For this review, take the finished solid that the model builds, in its own axes (mm). Coordinates: 2 decimals unless noted, no trailing zeros. Write each loop counter-clockwise with the first axis right and the second up, starting at its lowest first coordinate (ties: lowest second). Pieces come first, ordered by that corner, then holes.
1) We need section B-B on z = 1.9. Give the number of separate pieces and of enclosed holes in the cut face, then the cut area to 3 significant figures.
2) We need section A-A on x = -457. Write out the cut boundary in (y, z).
3) We need section C-C on x = -710.5. Write out the cut boundary in (y, z).
4) To check wall thickness, follow line 1 along X through (y, z) = (-180, 2.1); line 2 along Y through (x, z) = (-730, 1.8); line 3 along X through (y, z) = (20.5, 2.3). State the ranges of each line that lie inside material, in increasing order.
5) Insertion check: P1, Ø3.5, axis at x = -635, y = 15, coming from the +Z side; P2, Ø1.5, axis at x = -378.5, z = 2.5, coming from the -Y side. Each pin has a flat end and moves straight along its axis. Give the tip position at first contact, or say it passes through.
from build123d import *

# Parameters (mm, degrees)
F0_W     = 60
F0_H     = 160
F1_DEPTH = 3
F2_R     = 2.05
F3_DEPTH = 3
F4_W     = 720
F4_H     = 60
F4_R     = 2.05
F5_DEPTH = 3
F6_W     = 130
F6_H     = 30
F7_DEPTH = 25


with BuildPart() as f1:
    # F0 (on Top) → F1 (new body)
    with BuildSketch(Plane.XY):
        with Locations((30, -110)):
            Rectangle(F0_W, F0_H)
        Polygon((0, -30), (60, -30), (60, 30), (-60, 30), (-60, -30), align=None)
    extrude(amount=F1_DEPTH)

    # F2 (on face) → F3 (cut)
    with BuildSketch(Plane.XY.offset(3)):
        with BuildLine():
            Line((-50.5, 11.5), (-39.5, 11.5))
            ThreePointArc((-39.5, 11.5), (-36, 15), (-39.5, 18.5))
            Line((-39.5, 18.5), (-50.5, 18.5))
            ThreePointArc((-50.5, 18.5), (-54, 15), (-50.5, 11.5))
        make_face()
        with BuildLine():
            ThreePointArc((-20.5, 18.5), (-24, 15), (-20.5, 11.5))
            Line((-20.5, 11.5), (-9.5, 11.5))
            ThreePointArc((-9.5, 11.5), (-6, 15), (-9.5, 18.5))
            Line((-9.5, 18.5), (-20.5, 18.5))
        make_face()
        with BuildLine():
            ThreePointArc((-50.5, -11.5), (-54, -15), (-50.5, -18.5))
            Line((-50.5, -18.5), (-39.5, -18.5))
            ThreePointArc((-39.5, -18.5), (-36, -15), (-39.5, -11.5))
            Line((-39.5, -11.5), (-50.5, -11.5))
        make_face()
        with BuildLine():
            ThreePointArc((-20.5, -11.5), (-24, -15), (-20.5, -18.5))
            Line((-20.5, -18.5), (-9.5, -18.5))
            ThreePointArc((-9.5, -18.5), (-6, -15), (-9.5, -11.5))
            Line((-9.5, -11.5), (-20.5, -11.5))
        make_face()
        with BuildLine():
            ThreePointArc((41.5, -165.5), (45, -169), (48.5, -165.5))
            Line((48.5, -165.5), (48.5, -154.5))
            ThreePointArc((48.5, -154.5), (45, -151), (41.5, -154.5))
            Line((41.5, -154.5), (41.5, -165.5))
        make_face()
        with BuildLine():
            ThreePointArc((11.5, -165.5), (15, -169), (18.5, -165.5))
            Line((18.5, -165.5), (18.5, -154.5))
            ThreePointArc((18.5, -154.5), (15, -151), (11.5, -154.5))
            Line((11.5, -154.5), (11.5, -165.5))
        make_face()
        with Locations((15, -180)):
            Circle(F2_R)
        with Locations((45, -180)):
            Circle(F2_R)
        with Locations((15, -135)):
            Circle(F2_R)
        with Locations((45, -135)):
            Circle(F2_R)
        with BuildLine():
            ThreePointArc((41.5, 9.5), (45, 6), (48.5, 9.5))
            Line((48.5, 9.5), (48.5, 20.5))
            ThreePointArc((48.5, 20.5), (45, 24), (41.5, 20.5))
            Line((41.5, 20.5), (41.5, 9.5))
        make_face()
        with BuildLine():
            ThreePointArc((11.5, 9.5), (15, 6), (18.5, 9.5))
            Line((18.5, 9.5), (18.5, 20.5))
            ThreePointArc((18.5, 20.5), (15, 24), (11.5, 20.5))
            Line((11.5, 20.5), (11.5, 9.5))
        make_face()
        with Locations((15, -25)):
            Circle(F2_R)
        with Locations((45, -25)):
            Circle(F2_R)
        with Locations((45, -80)):
            Circle(F2_R)
        with Locations((15, -80)):
            Circle(F2_R)
    extrude(amount=-F3_DEPTH, mode=Mode.SUBTRACT)

    # F4 (on face) → F5 (join)
    with BuildSketch(Plane(origin=(0, 0, 0), x_dir=(1, 0, 0), z_dir=(0, 0, -1))):
        with Locations((-420, 0)):
            Rectangle(F4_W, F4_H)
        with BuildLine():
            ThreePointArc((-759.5, -11.5), (-756, -15), (-759.5, -18.5))
            Line((-759.5, -18.5), (-770.5, -18.5))
            ThreePointArc((-770.5, -18.5), (-774, -15), (-770.5, -11.5))
            Line((-770.5, -11.5), (-759.5, -11.5))
        make_face(mode=Mode.SUBTRACT)
        with Locations((-730, -15)):
            Circle(F4_R, mode=Mode.SUBTRACT)
        with Locations((-680, -15)):
            Circle(F4_R, mode=Mode.SUBTRACT)
        with Locations((-635, -15)):
            Circle(F4_R, mode=Mode.SUBTRACT)
        with Locations((-395, -15)):
            Circle(F4_R, mode=Mode.SUBTRACT)
        with Locations((-155, -15)):
            Circle(F4_R, mode=Mode.SUBTRACT)
        with Locations((-110, -15)):
            Circle(F4_R, mode=Mode.SUBTRACT)
        with BuildLine():
            ThreePointArc((-759.5, 18.5), (-756, 15), (-759.5, 11.5))
            Line((-759.5, 11.5), (-770.5, 11.5))
            ThreePointArc((-770.5, 11.5), (-774, 15), (-770.5, 18.5))
            Line((-770.5, 18.5), (-759.5, 18.5))
        make_face(mode=Mode.SUBTRACT)
        with Locations((-730, 15)):
            Circle(F4_R, mode=Mode.SUBTRACT)
        with Locations((-680, 15)):
            Circle(F4_R, mode=Mode.SUBTRACT)
        with Locations((-635, 15)):
            Circle(F4_R, mode=Mode.SUBTRACT)
        with Locations((-395, 15)):
            Circle(F4_R, mode=Mode.SUBTRACT)
        with Locations((-155, 15)):
            Circle(F4_R, mode=Mode.SUBTRACT)
        with Locations((-110, 15)):
            Circle(F4_R, mode=Mode.SUBTRACT)
    extrude(amount=-F5_DEPTH)

    # F6 (on face) → F7 (cut)
    with BuildSketch(Plane(origin=(0, 0, 0), x_dir=(1, 0, 0), z_dir=(0, 0, -1))):
        with Locations((-515, 0)):
            Rectangle(F6_W, F6_H)
        with Locations((-275, 0)):
            Rectangle(F6_W, F6_H)
    extrude(amount=-F7_DEPTH, mode=Mode.SUBTRACT)


solid = f1.part
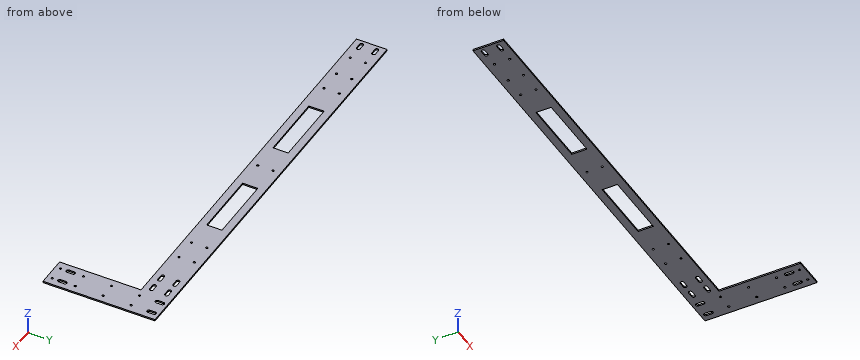
Result:
1. separate pieces: 1
1. enclosed holes: 32
1. area: 50,800 mm2
2. outline: (-30, 0) - (-15, 0) - (-15, 3) - (-30, 3) - close; (15, 0) - (30, 0) - (30, 3) - (15, 3) - close
3. outline: (-30, 0) - (30, 0) - (30, 3) - (-30, 3) - close
4. line 1: x = 0 to 12.95, 17.05 to 42.95, 47.05 to 60
4. line 2: y = -30 to -17.05, -12.95 to 12.95, 17.05 to 30
4. line 3: x = -780 to 11.5, 18.5 to 41.5, 48.5 to 60
5. P1: passes through
5. P2: stops at y = -30
